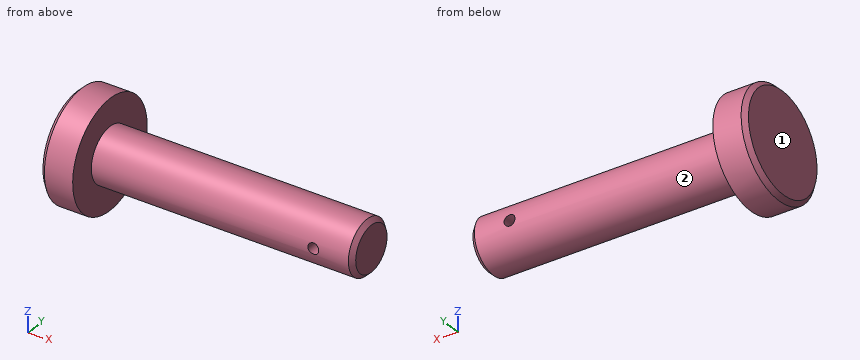
```python
from build123d import *

# Parameters (mm, degrees)
F2_DEPTH = 25.4
F3_SIZE  = 2.54


with BuildPart() as f1:
    # F0 (on Front) → F1 (revolve)
    with BuildSketch(Plane.XZ):
        with BuildLine():
            Line((-76.2, 15.875), (-76.2, 0))
            Line((-76.2, 0), (50.0140764832, 0))
            ThreePointArc((50.0140764832, 0), (53.1890764832, 3.175), (56.3640764832, 0))
            Line((56.3640764832, 0), (76.2, 0))
            Line((76.2, 0), (76.2, 15.875))
            Line((76.2, 15.875), (-76.2, 15.875))
        make_face()
        Polygon((-95.25, 0), (-76.2, 0), (-76.2, 15.875), (-76.2, 31.75), (-95.25, 31.75), align=None)
    revolve(axis=Axis((-9.525, 0, 0), (-1, 0, 0)))

    # F0 (on Front) → F2 (cut, symmetric)
    with BuildSketch(Plane.XZ):
        with BuildLine():
            Line((56.3640764832, 0), (50.0140764832, 0))
            ThreePointArc((50.0140764832, 0), (53.1890764832, -3.175), (56.3640764832, 0))
        make_face()
        with BuildLine():
            ThreePointArc((56.3640764832, 0), (53.1890764832, 3.175), (50.0140764832, 0))
            Line((50.0140764832, 0), (56.3640764832, 0))
        make_face()
    extrude(amount=F2_DEPTH, both=True, mode=Mode.SUBTRACT)

    # F3
    f3_edges = [f1.edges().sort_by_distance(p)[0] for p in [
        (76.2, 0, -15.875),
        (-95.25, 0, -31.75),
    ]]
    chamfer(f3_edges, length=F3_SIZE)


solid = f1.part
```
Input: part model. Units: mm. Frame: model coordinates. Face numbers are marked on the shaded views. A direction names the side the tool comes from. Give positions to 0.01 mm unless a question says otherwise; leave off trailing zeros. Order: outer loops, then holes, each group sorted by start corner. A loop starts at its lowest first (then second) coordinate and runs counter-clockwise, first axis right, second up. Notation, with made-up numbers: (45.5, 70.25) - (96.5, 70.25) arc R22 cw to (96.5, 89.25) - close; hole circle Ø8 at (71.25, 29). An arc over 180 degrees is marked (long way). Put each result on its own line as item: value.
Item 1: Section query B-B, the plane z = 0. Return loops of the section in (x, y) (3 decimals).
Found:
outline: (-95.25, -29.21) - (-92.71, -31.75) - (-76.2, -31.75) - (-76.2, -15.875) - (50.014, -15.875) - (50.014, 15.875) - (-76.2, 15.875) - (-76.2, 31.75) - (-92.71, 31.75) - (-95.25, 29.21) - close; (56.364, -15.875) - (73.66, -15.875) - (76.2, -13.335) - (76.2, 13.335) - (73.66, 15.875) - (56.364, 15.875) - close
Item 2: Section query A-A, the plane y = 0. Return loops of the section in (x, z) (3 decimals), then the cut area to 3 significant figures.
Found:
outline: (-95.25, -29.21) - (-92.71, -31.75) - (-76.2, -31.75) - (-76.2, -15.875) - (73.66, -15.875) - (76.2, -13.335) - (76.2, 13.335) - (73.66, 15.875) - (-76.2, 15.875) - (-76.2, 31.75) - (-92.71, 31.75) - (-95.25, 29.21) - close; hole circle Ø6.35 at (53.189, 0)
area: 6,000 mm^2
Item 3: Section query C-C, the plane x = -13.5. Return loops of the section in (y, z) (3 decimals).
Found:
outline: circle Ø31.75 at (0, 0)
Item 4: Ray query, L1, parallel to X at y = 5, z = 0; L2, parallel to X at y = 3, z = -23; L3, parallel to Y at x = -45, z = 1. Return the intervals inside material, ascending. Write a range as from..to.
Found:
L1: x = -95.25..50.01, 56.36..76.2
L2: x = -95.25..-76.2
L3: y = -15.84..15.84
Item 5: Access query for the marked faces 1 and 2. Directions: +Z, -Z, +X, -X, +Y, -Y. A direction counts if a zero-diameter tool reaches every point of the face in a straight line with its end or side. Return the directions, or none.
Found:
face 1: +Z, -Z, -X, +Y, -Y
face 2: +X
Item 6: Contact query for flat-ended pins moving along their axis: pin 1 (12 mm diameter, centred on x = -48.5, z = -24.5, fed in from +Y); pin 2 (10 mm diameter, centred on x = 53.19, z = 0, fed in from -Y) (3 decimals); pin 3 (3 mm diameter, centred on x = -59, y = 14, fed in from -Z); pin 4 (6 mm diameter, centred on x = 26.5, z = -15.5, fed in from -Y). Output: stop coordinate, or through.
Found:
pin 1: passes through
pin 2: stops at y = -15.875
pin 3: stops at z = -9.79
pin 4: stops at y = -9.79
